from build123d import *

# Parameters (mm, degrees)
F1_DEPTH = 50.8
F2_W     = 50.8
F2_H     = 12.7
F3_DEPTH = 2.54


with BuildPart() as f1:
    # F0 (on Right) → F1 (new body)
    with BuildSketch(Plane.YZ):
        Polygon((-97.119585, 21.958653), (-101.6, 18.928962), (-101.6, 0), (0, 0), (0, 87.63165), align=None)
        Polygon((-101.6, 42.036834), (-101.6, 18.928962), (-97.119585, 21.958653), (-97.119585, 42.036834), align=None)
    extrude(amount=F1_DEPTH)

    # F2 (on face) → F3 (join)
    with BuildSketch(Plane(origin=(0, -40.663519, 60.134671), x_dir=(1, 0, 0), z_dir=(0, -0.56016, 0.828385))):
        with Locations((25.4, 21.767601)):
            Rectangle(F2_W, F2_H)
    extrude(amount=F3_DEPTH)


solid = f1.part
Read the model definition and answer for the solid it produces. Units are mm, in the model's axes. A direction names the side the tool comes from. Give positions to 0.01 mm unless a question says otherwise; leave off trailing zeros. Write each loop counter-clockwise with the first axis right and the second up, starting at its lowest first coordinate (ties: lowest second). Pieces come first, ordered by that corner, then holes. Notation, with made-up numbers: (40, 23) - (73, 23) arc R18 ccw to (73, 34) - close; hole circle Ø3 at (11.25, 89). An arc over 180 degrees is marked (long way). Answer in a Markdown table with one row per item. Add a question column.
Item 1: Determine the mould class of faces 1 (the face through (25, -52, 0)), 2 (the face through (25, -101.6, 21)), 3 (the face through (25.044, -62.021, 45.693)) for opening direction Y: pulls with the +Y half, pulls with the -Y half, needs draft (parallel to the pull), parting line crosses it, or undercut.
Item 2: Section A-A, the plane z = 39 is taken. Write down the section's boundary in (x, y), and give its area (3 significant figures).
Item 3: Section C-C, the plane y = -86 is taken. Write down the section's boundary in (x, z).
Item 4: Section B-B, the plane x = 38 is taken. Write down the section's boundary in (y, z).
Item 5: Flat-ended cylindrical pins translate along their axes: P1, Ø5, axis at x = 35.5, y = -99.5, coming from the +Z side; P2, Ø8, axis at x = 35.5, y = -54.5, coming from the +Z side; P3, Ø10, axis at x = 28, y = -82, coming from the +Z side. Find the tip coordinate at first contact, or state that the pin passes through.
Item 6: A tool of negligible diameter and unlimited length cuts with its end or side. For faces 4 (the face through (0, -40, 35)), 5 (the face through (25, -99, 42.037)), 6 (the face through (25, -97.12, 32)), from which of +Z, -Z, +X, -X, +Y, -Y can it reach the whole face along a straight path? Write none if from no direction.
Item 7: Section D-D, the plane z = 48.5 is taken. Write down the section's boundary in (x, y).
Item 8: Find the intervals of material crossed by L1, parallel to Y at x = 40, z = 39; L2, parallel to Y at x = 46, z = 41; L3, parallel to Z at x = 25, y = -58, in increasing order.
Recorded:
| question | item | result |
|---|---|---|
| 1 | face 1 | needs draft |
| 1 | face 2 | pulls with the -Y half |
| 1 | face 3 | undercut |
| 2 | outline | (0, -101.6) - (50.8, -101.6) - (50.8, -97.12) - (0, -97.12) - close; (0, -71.92) - (50.8, -71.92) - (50.8, 0) - (0, 0) - close |
| 2 | area | 3,880 mm2 |
| 3 | outline | (0, 0) - (50.8, 0) - (50.8, 29.48) - (0, 29.48) - close |
| 4 | outline | (-101.6, 0) - (0, 0) - (0, 87.63) - (-17.37, 75.89) - (-18.79, 77.99) - (-29.31, 70.88) - (-27.89, 68.77) - (-97.12, 21.96) - (-97.12, 42.04) - (-101.6, 42.04) - close |
| 5 | P1 | stops at z = 42.04 |
| 5 | P2 | stops at z = 53.48 |
| 5 | P3 | stops at z = 35.56 |
| 6 | face 4 | +Z, -Z, -X, +Y, -Y |
| 6 | face 5 | +Z, +X, -X, -Y |
| 6 | face 6 | +Z, +X, -X |
| 7 | outline | (0, -57.87) - (50.8, -57.87) - (50.8, 0) - (0, 0) - close |
| 8 | L1 | y = -101.6 to -97.12, -71.92 to 0 |
| 8 | L2 | y = -101.6 to -97.12, -68.96 to 0 |
| 8 | L3 | z = 0 to 48.41 |
